Autodesk Inventor part; units mm, degrees
ref_plane "YZ Plane" through (0, 0, 0) normal (1, 0, 0) x (0, 1, 0)
ref_plane "XZ Plane" through (0, 0, 0) normal (0, 1, 0) x (-1, 0, 0)
ref_plane "XY Plane" through (0, 0, 0) normal (0, 0, 1) x (1, 0, 0)
sketch "Sketch1" plane through (0, 0, 0) normal (0, 1, 0) x (-1, 0, 0)
  circle A0 centre (0, 0) radius 41
  circle A1 centre (0, 0) radius 12.5
  dimension "d0" = 82
  dimension "d1" = 25
extrude "Extrusion1" add sketch "Sketch1" along normal blind 2
sketch "Sketch2" plane through (0, 2, 0) normal (0, 1, 0) x (1, 0, 0)
  line L0 (0, 0) -> (0, -19)
  line L1 (0, 0) -> (19, 0) construction
  circle A0 centre (0, -19) radius 2.5
  dimension "d4" = 19
  dimension "d5" = 90
  dimension "d6" = 5
extrude "Extrusion2" add sketch "Sketch2" along normal blind 14
sketch "Sketch3" plane through (0, 16, 19) normal (0, 1, 0) x (1, 0, 0)
  circle A0 centre (0, 0) radius 2.5
  circle A1 centre (0, 0) radius 1
  point P0 (0, 19)
  dimension "d9" = 2
extrude "Extrusion3" cut sketch "Sketch3" against normal blind 14 contours A1
sketch "Sketch4" plane through (0, 16, 19) normal (0, 1, 0) x (1, 0, 0)
  circle A0 centre (0, 0) radius 1
  line L0 (0, 0) -> (0, 2.5)
  circle A1 centre (0, 0) radius 2.5
  line L1 (0, 2.5) -> (0, 2)
  line L2 (0, 2) -> (-3, 2)
  line L3 (-3, 2) -> (-3, 2.5)
  line L4 (-3, 2.5) -> (0, 2.5)
  line L5 (0, 2.5) -> (0, 2)
  line L6 (0, 2) -> (3, 2)
  line L7 (3, 2) -> (3, 2.5)
  line L8 (3, 2.5) -> (0, 2.5)
  point P0 (0, 19)
  point P1 (-1.5, 2)
  dimension "d12" = 0.5
  dimension "d13" = 3
  dimension "d14" = 0.5
  dimension "d15" = 3
extrude "Extrusion4" cut sketch "Sketch4" against normal blind 14 contours L2 A1 L0 | L0 A1 L6 | L8 L7 L6 A1
properties part number "lid"
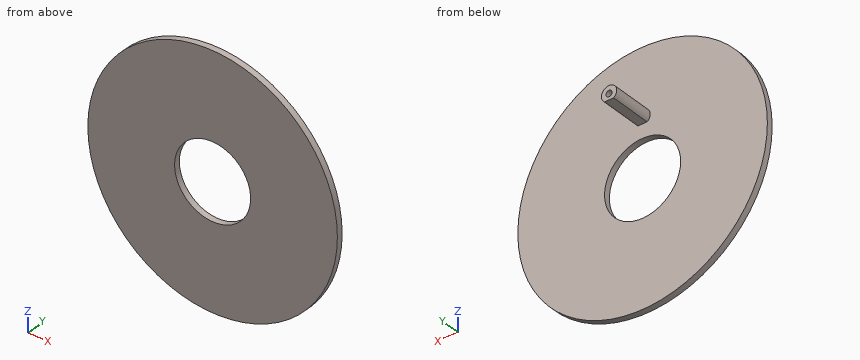
Could you check a few things on this model? Use its own coordinates, in mm. Give positions to 0.01 mm unless a question says otherwise; leave off trailing zeros. Order: outer loops, then holes, each group sorted by start corner. A loop starts at its lowest first (then second) coordinate and runs counter-clockwise, first axis right, second up. Notation, with made-up numbers: (20, 50) - (42, 50) arc R3 cw to (42, 55) - close; hole circle Ø4 at (78.5, 71). An arc over 180 degrees is marked (long way). Return JSON: item names as keys, results as strings. Group by question number.
Q1. Will these pins go through, and if not, where does the flat tip stop? pin 1 Ø5 at (y, z) = (6.5, -6) entering from -X; pin 2 Ø3.5 at (x, y) = (-0.5, 6) entering from -Z; pin 3 Ø10 at (x, z) = (19.5, 12) entering from +Y.
Q2. Suppose I cut it at C-C, the plane y = 7.75. Please give me the cut outline in (x, z), and give its area (3 significant figures).
Q3. Suppose I cut it at A-A, the plane x = 0. Please give me the cut outline in (y, z).
Q4. Suppose I cut it at B-B, the plane z = 0. Please give me the cut outline in (x, y), and give its area (3 significant figures).
Q5. Suppose I cut it at D-D, the plane z = 9. Please give me the cut outline in (x, y).
Q6. Please list where these lines run through material, in increasing order: line 1 along X through (y, z) = (8, 19); line 2 along Z through (x, y) = (0, 1.5); line 3 along Y through (x, z) = (-16, 1.5). Write a range as [from, to].
Resolved:
{
 "1": {"pin 1": "passes through", "pin 2": "stops at z = 17", "pin 3": "stops at y = 2"},
 "2": {"outline": "(-1.5, 17) - (1.5, 17) arc R2.5 ccw (long way) to start; hole circle Ø2 at (0, 19)", "area": "15.5 mm2"},
 "3": {"outline": "(0, -41) - (2, -41) - (2, -12.5) - (0, -12.5) - close; (0, 12.5) - (2, 12.5) - (2, 17) - (16, 17) - (16, 18) - (2, 18) - (2, 20) - (16, 20) - (16, 21.5) - (2, 21.5) - (2, 41) - (0, 41) - close"},
 "4": {"outline": "(-41, 0) - (-12.5, 0) - (-12.5, 2) - (-41, 2) - close; (12.5, 0) - (41, 0) - (41, 2) - (12.5, 2) - close", "area": "114 mm2"},
 "5": {"outline": "(-40, 0) - (-8.67, 0) - (-8.67, 2) - (-40, 2) - close; (8.67, 0) - (40, 0) - (40, 2) - (8.67, 2) - close"},
 "6": {"line 1": "x = [-2.5, -1], [1, 2.5]", "line 2": "z = [-41, -12.5], [12.5, 41]", "line 3": "y = [0, 2]"}
}
